Autodesk Inventor part; units mm, degrees
ref_plane "YZ Plane" through (0, 0, 0) normal (1, 0, 0) x (0, 1, 0)
ref_plane "XZ Plane" through (0, 0, 0) normal (0, 1, 0) x (-1, 0, 0)
ref_plane "XY Plane" through (0, 0, 0) normal (0, 0, 1) x (1, 0, 0)
sketch "Sketch1" plane through (0, 0, 0) normal (0, 1, 0) x (-1, 0, 0)
  circle A0 centre (-21.92, 0) radius 1.75
  circle A1 centre (21.92, 0) radius 1.75
  circle A2 centre (0, 0) radius 18.13
  circle A3 centre (-21.92, 0) radius 3.715
  circle A4 centre (21.92, 0) radius 3.715
  line L0 (-25.635, 0) -> (-25.635, -14)
  line L1 (-25.635, -14) -> (-11.5194, -14)
  line L2 (11.5194, -14) -> (25.635, -14)
  line L3 (25.635, -14) -> (25.635, 0)
  line L4 (24.0715, 3.0286) -> (15.7877, 8.9132)
  line L5 (-24.0715, 3.0286) -> (-15.7877, 8.9132)
  dimension "d0" = 3.5
  dimension "d1" = 43.84
  dimension "d2" = 21.92
  dimension "d3" = 36.26
  dimension "d4" = 51.27
  dimension "d5" = 14
  dimension "d7" = 35.389
extrude "Extrusion1" add sketch "Sketch1" along normal blind 1.6
properties part number "Mellow Fly SHT36" material "Copper, Alloy"
Read the model definition and answer for the solid it produces. Units are mm, in the model's axes. A direction names the side the tool comes from. Round coordinates to 2 decimals unless told otherwise and drop trailing zeros. Write each loop counter-clockwise with the first axis right and the second up, starting at its lowest first coordinate (ties: lowest second). Pieces come first, ordered by that corner, then holes.
Q1. Find section B-B on x = -21.92. Determine the outline of the cut face in (y, z).
Values:
outline: (0, -14) - (1.6, -14) - (1.6, -1.75) - (0, -1.75) - close; (0, 1.75) - (1.6, 1.75) - (1.6, 4.56) - (0, 4.56) - close
Q2. Find section D-D on x = 9. Determine the outline of the cut face in (y, z), and give its area (3 significant figures).
Values:
outline: (0, -15.74) - (1.6, -15.74) - (1.6, 15.74) - (0, 15.74) - close
area: 50.4 mm2
Q3. A tool of negligible diameter and unlimited length cuts with its end or side. For faces 1 (the face through (19, 1, -14)), 2 (the face through (-20.53, 0.79, 1.06)), 3 (the face through (-18, 1, -14)), from which of +Z, -Z, +X, -X, +Y, -Y can it reach the whole face along a straight path? Write none if from no direction.
Values:
face 1: -Z, +X, +Y, -Y
face 2: +Y, -Y
face 3: -Z, -X, +Y, -Y
Q4. Straight lines are drawn through the part: line 1 (X direction, y = 0.55, z = 1); line 2 (X direction, y = 1.25, z = 0.5); line 3 (Z direction, x = 23, y = 0.2). For each, find the intervals that lie inside material, in ascending order.
Values:
line 1: x = -25.5 to -23.36, -20.48 to 20.48, 23.36 to 25.5
line 2: x = -25.6 to -23.6, -20.24 to 20.24, 23.6 to 25.6
line 3: z = -14 to -1.38, 1.38 to 3.79
Q5. Find section A-A on y = 0.4. State how many separate pieces and enclosed holes the cut face has, and give its area (3 significant figures).
Values:
separate pieces: 1
enclosed holes: 2
area: 1,360 mm2
Q6. Find section C-C on z = 15. Determine the outline of the cut face in (x, y).
Values:
outline: (-10.18, 0) - (10.18, 0) - (10.18, 1.6) - (-10.18, 1.6) - close
Q7. The mould has two halves that part along X. Classify faces 4 (the face through (20.251, 0.789, -0.526)), 5 (the face through (-19.99, 0.79, 5.93)), 6 (the face through (19.99, 0.79, 5.93)): released by +X, released by -X, zero draft, split by the parting line, or undercut.
Values:
face 4: undercut
face 5: released by -X
face 6: released by +X
